```python
from build123d import *

# Parameters (mm, degrees)
SKETCH1_R           = 1.45
BOSS_EXTRUDE1_DEPTH = 4
SKETCH2_R           = 5.35614303
CUT_EXTRUDE1_DEPTH  = 1.4
CUT_EXTRUDE1_TAPER  = 11
CUT_EXTRUDE2_DEPTH  = 5.5


with BuildPart() as part:
    # Sketch1 → Boss-Extrude1 (new body)
    with BuildSketch(Plane.XY):
        with BuildLine():
            Line((-19, 6.631961257), (-19, 13.975))
            ThreePointArc((-19, 13.975), (-14.5, 18.475), (-10, 13.975))
            Line((-10, 13.975), (-10, -13.975))
            ThreePointArc((-10, -13.975), (-14.5, -18.475), (-19, -13.975))
            Line((-19, -13.975), (-19, -6.651961257))
            ThreePointArc((-19, -6.651961257), (-22.522820535, -0.01), (-19, 6.631961257))
        make_face()
        with Locations((-14.5, -13.975)):
            Circle(SKETCH1_R, mode=Mode.SUBTRACT)
        with Locations((-14.5, 13.975)):
            Circle(SKETCH1_R, mode=Mode.SUBTRACT)
    extrude(amount=BOSS_EXTRUDE1_DEPTH)

    # Sketch2 → Cut-Extrude1 (cut)
    with BuildSketch(Plane(origin=(0, 0, 0), x_dir=(-1, 0, 0), z_dir=(0, 0, -1))):
        with Locations((14.5, -0.01)):
            Circle(SKETCH2_R)
    extrude(amount=-CUT_EXTRUDE1_DEPTH, taper=CUT_EXTRUDE1_TAPER, mode=Mode.SUBTRACT)

    # Sketch3 → Cut-Extrude2 (cut)
    with BuildSketch(Plane.XY.offset(4)):
        with BuildLine():
            Line((-14.5, -2.270184411), (-10, -2.270184411))
            Line((-10, -2.270184411), (-10, 2.250184411))
            Line((-10, 2.250184411), (-14.5, 2.250184411))
            ThreePointArc((-14.5, 2.250184411), (-16.760184411, -0.01), (-14.5, -2.270184411))
        make_face()
    extrude(amount=-CUT_EXTRUDE2_DEPTH, mode=Mode.SUBTRACT)


solid = part.part
```
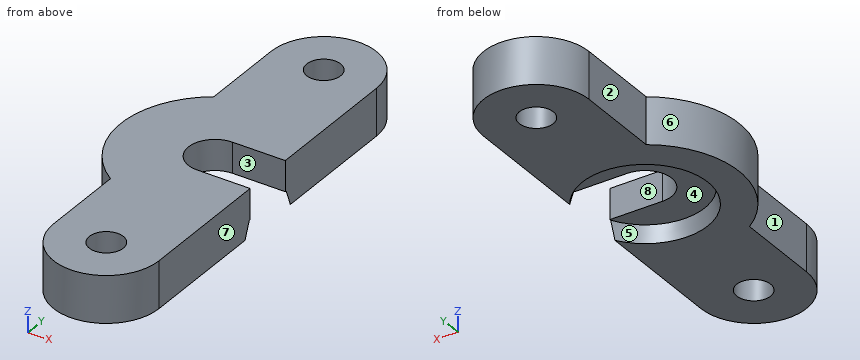
Check sheet for the modelled part. Datum: model origin and axes. Units: mm. Face numbers are marked on the shaded views. A direction names the side the tool comes from. Give positions to 0.01 mm unless a question says otherwise; leave off trailing zeros. Loops run counter-clockwise (first coordinate to the right, second up) from the corner with the lowest first, then second, coordinate; pieces in that order, holes last. Notation, with made-up numbers: (-40, 25) - (-34, 25) arc R25 cw to (-34, 61) - close; hole circle Ø4 at (67.5, -0.75). An arc over 180 degrees is marked (long way). One line per question, with ' | ' between items. Start each with the question number.
1. Cross-section at C-C, the plane y = -0.01. Enter the section's corners in (x, z).
2. Gauge pin test, flat ends, axial feed: pin 1 Ø0.8 at (x, z) = (-12.5, 2) entering from +Y; pin 2 Ø0.8 at (x, z) = (-13.5, 3) entering from -Y; pin 3 Ø2 at (x, y) = (-16, -1) entering from -Z. Record the tip position at first contact, or that the pin passes through.
3. Cross-section at D-D, the plane y = -7. Enter the section's corners in (x, z).
4. Cross-section at A-A, the plane z = 2.1. Enter the section's corners in (x, y) (3 decimals).
5. Material ranges on line 1 along Y through (x, z) = (-14.5, 2) (3 decimals); line 2 along X through (y, z) = (-14, 3.5); line 3 along X through (y, z) = (-8, 0.65), recorded low to high. Write a range as [from, to].
6. Set-up check for the marked faces 1, 2, 3 and 4: record each of +Z, -Z, +X, -X, +Y, -Y from which the full face is reachable in a straight line by a thin tool's end or side.
7. Cross-section at B-B, the plane y = 13. Enter the section's corners in (x, z).
8. Draft check along Y on the marked faces 5, 6, 7 and 8. Enter one of: released by +Y, released by -Y, zero draft, split by the parting line, or undercut.
Check result:
1) outline: (-22.52, 0) - (-19.86, 0) - (-19.58, 1.4) - (-16.76, 1.4) - (-16.76, 4) - (-22.52, 4) - close
2) pin 1: stops at y = 18.18 | pin 2: stops at y = -18.43 | pin 3: stops at z = 1.4
3) outline: (-19, 0) - (-10, 0) - (-10, 4) - (-19, 4) - close
4) outline: (-19, -13.975) arc R4.5 ccw to (-10, -13.975) - (-10, -2.27) - (-14.5, -2.27) arc R2.26 cw to (-14.5, 2.25) - (-10, 2.25) - (-10, 13.975) arc R4.5 ccw to (-19, 13.975) - (-19, 6.632) arc R8.023 ccw to (-19, -6.652) - close; hole circle Ø2.9 at (-14.5, -13.975); hole circle Ø2.9 at (-14.5, 13.975)
5) line 1: y = [-18.475, -15.425], [-12.525, -2.27], [2.25, 12.525], [15.425, 18.475] | line 2: x = [-19, -15.95], [-13.05, -10] | line 3: x = [-19, -10]
6) face 1: +Z, -Z, -X, -Y | face 2: +Z, -Z, -X, +Y | face 3: +Z, -Z, +X | face 4: -Z
7) outline: (-19, 0) - (-15.57, 0) - (-15.57, 4) - (-19, 4) - close; (-13.43, 0) - (-10, 0) - (-10, 4) - (-13.43, 4) - close
8) face 5: undercut | face 6: split by the parting line | face 7: zero draft | face 8: undercut
